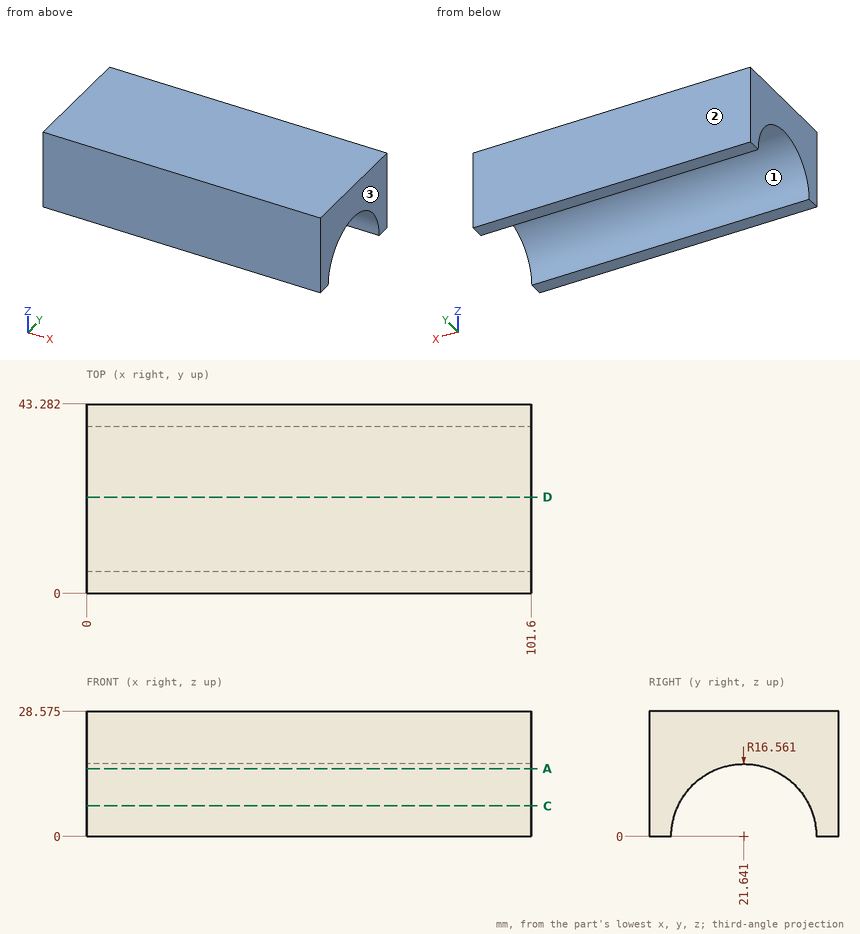
Verification items for this drawing (mm, ordinates from the low corner). Give positions to 0.01 mm unless a question says otherwise; leave off trailing zeros. Loops run counter-clockwise (first coordinate to the right, second up) from the corner with the lowest first, then second, coordinate; pieces in that order, holes last. Notation, with made-up numbers: M 43,37.25 L 84,37.25 A15 ccw 84,60.25 Z; hole C -8.5,79.25 d7. An arc over 180 degrees is marked long. Write each question's results on one line, items separated by ' | '.
1) Section check A-A, the plane z = 15.5. Record the boundary of the cut face in (x, y), plus the area to 3 significant figures.
Answers follow:
outline: M 0,0 L 101.6,0 L 101.6,15.81 L 0,15.81 Z; M 0,27.47 L 101.6,27.47 L 101.6,43.28 L 0,43.28 Z | area: 3,210 mm2
2) Gauge pin test, flat ends, axial feed: pin 1 (3 mm diameter, centred on x = 51, y = 29, fed in from -Z); pin 2 (3 mm diameter, centred on x = 66.5, y = 26, fed in from -Z). Record the tip position at first contact, or that the pin passes through.
Answers follow:
pin 1: z = 13.99 | pin 2: z = 15.49
3) Section check D-D, the plane y = 22. Record the boundary of the cut face in (x, z) (1 decimal), plus the area to 3 significant figures.
Answers follow:
outline: M 0,16.6 L 101.6,16.6 L 101.6,28.6 L 0,28.6 Z | area: 1,220 mm2
4) Section check C-C, the plane z = 7. Record the boundary of the cut face in (x, y).
Answers follow:
outline: M 0,0 L 101.6,0 L 101.6,6.63 L 0,6.63 Z; M 0,36.65 L 101.6,36.65 L 101.6,43.28 L 0,43.28 Z
5) Thickness scan on line 1 (Y direction, x = 44, z = 6.25) (1 decimal); line 2 (Y direction, x = 44.5, z = 10); line 3 (Z direction, x = 76, y = 22) (1 decimal). Record the ranges inside material, lowest first.
Answers follow:
line 1: 0 to 6.3, 37 to 43.3 | line 2: 0 to 8.44, 34.84 to 43.28 | line 3: 16.6 to 28.6
6) Release check for a two-part mould opening along Y. For the marked faces 1, 2 and 3 record: +Y half, -Y half, draft (parallel to the pull), parting line (faces both ways), or undercut.
Answers follow:
face 1: undercut | face 2: +Y half | face 3: draft
